The drawing under review shows one solid part. Ordinate dimensions are in mm from its lowest x, y, z. A direction names the side the tool comes from. Round coordinates to 2 decimals unless told otherwise and drop trailing zeros. Order: outer loops, then holes, each group sorted by start corner. A loop starts at its lowest first (then second) coordinate and runs counter-clockwise, first axis right, second up. Notation, with made-up numbers: M 59.5,-17.75 L 85.5,-17.75 A22 ccw 85.5,4.25 Z; hole C 26,-18 d10. An arc over 180 degrees is marked long. Answer as a JSON object with one key per item and string values. Group by question number.
1) Consider section A-A, the plane x = 10. Write out the cut boundary in (y, z), then the cut area to 3 significant figures.
2) For the marked faces 1 and 2, list the 3-axis set-ups (+Z, -Z, +X, -X, +Y, -Y) from which the entire face can be reached by the end or side of a thin tool; tool diameter is ignored.
3) To check wall thickness, follow line 1 (Y direction, x = 13.75, z = 1.75); line 2 (X direction, y = 0.5, z = 8); line 3 (Z direction, x = 8.5, y = 1). State the ranges of each line that lie inside material, in increasing order.
4) Consider section D-D, the plane x = 1.75. Write out the cut boundary in (y, z).
5) Consider section B-B, the plane z = 4.5. Write out the cut boundary in (x, y).
6) Consider section C-C, the plane y = 1.5. Write out the cut boundary in (x, z), then the cut area to 3 significant figures.
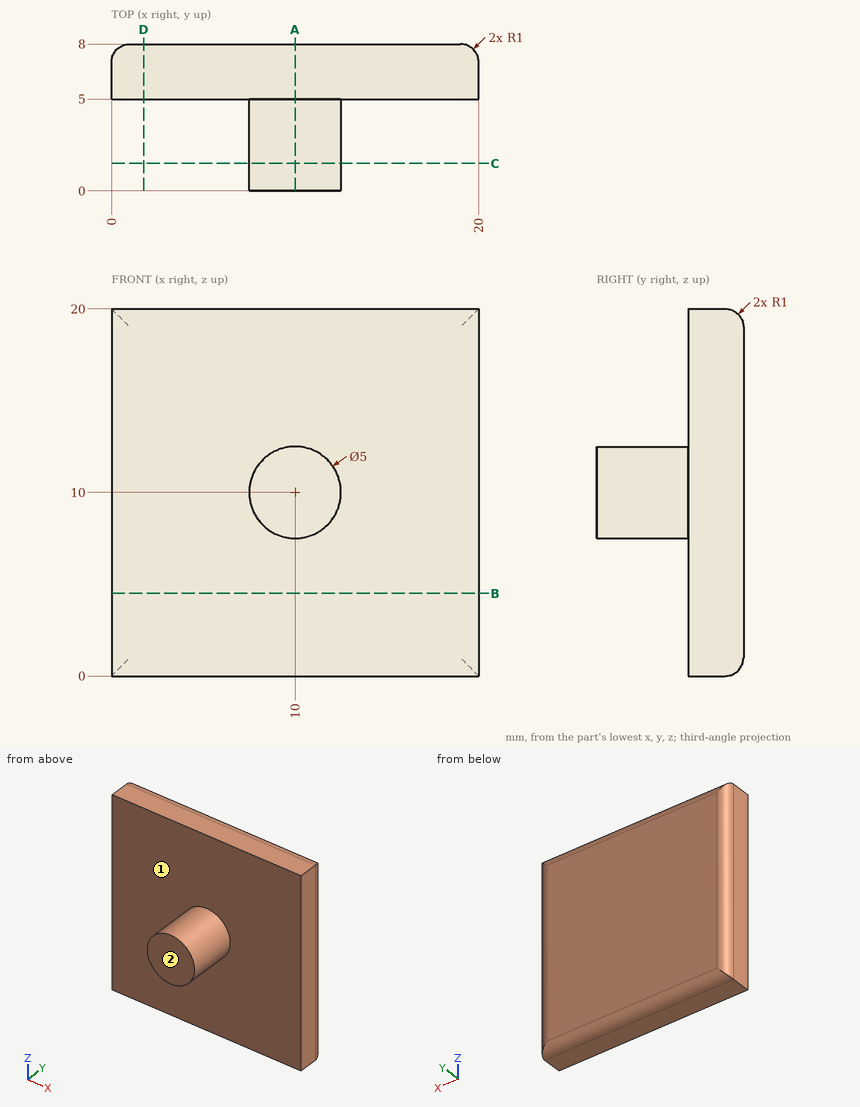
Results list:
{
 "1": {"outline": "M 0,7.5 L 5,7.5 L 5,0 L 7,0 A1 ccw 8,1 L 8,19 A1 ccw 7,20 L 5,20 L 5,12.5 L 0,12.5 Z", "area": "84.6 mm^2"},
 "2": {"face 1": "-Y", "face 2": "+Z, -Z, +X, -X, -Y"},
 "3": {"line 1": "5 to 8", "line 2": "8.5 to 11.5", "line 3": "8 to 12"},
 "4": {"outline": "M 5,0 L 7,0 A1 ccw 8,1 L 8,19 A1 ccw 7,20 L 5,20 Z"},
 "5": {"outline": "M 0,5 L 20,5 L 20,7 A1 ccw 19,8 L 1,8 A1 ccw 0,7 Z"},
 "6": {"outline": "C 10,10 d5", "area": "19.6 mm^2"}
}
